```python
from build123d import *

# Parameters (mm, degrees)
SKETCH1_R               = 15.25
SKETCH1_R_2             = 12.75
BOSS_EXTRUDE1_DEPTH     = 4
SKETCH2_R               = 15.25
SKETCH2_R_2             = 7.5
BOSS_EXTRUDE2_DEPTH     = 6
BOSS_EXTRUDE3_START     = -3
SKETCH3_R               = 15.25
BOSS_EXTRUDE3_DEPTH     = 3
SKETCH4_R               = 1.25
CUT_EXTRUDE1_DEPTH      = 10
CUT_EXTRUDE_THIN1_START = -70
CUT_EXTRUDE_THIN1_DEPTH = 25
SKETCH7_R               = 31
SKETCH7_R_2             = 26
BOSS_EXTRUDE4_DEPTH     = 5
CHAMFER3_SIZE           = 3
FILLET3_R               = 1
FILLET4_R               = 10


with BuildPart() as part:
    # Sketch1 → Boss-Extrude1 (new body)
    with BuildSketch(Plane(origin=(0, 0, 0), x_dir=(1, 0, 0), z_dir=(0, 1, 0))):
        with Locations(Location((0, 0, 0), (0, 0, 270))):
            Circle(SKETCH1_R)
        with Locations(Location((0, 0, 0), (0, 0, 270))):
            Circle(SKETCH1_R_2, mode=Mode.SUBTRACT)
    extrude(amount=BOSS_EXTRUDE1_DEPTH)

    # Sketch2 → Boss-Extrude2 (add)
    with BuildSketch(Plane(origin=(0, 4, 0), x_dir=(1, 0, 0), z_dir=(0, 1, 0))):
        with Locations(Location((0, 0, 0), (0, 0, 270))):
            Circle(SKETCH2_R)
        with Locations(Location((0, 0, 0), (0, 0, 270))):
            Circle(SKETCH2_R_2, mode=Mode.SUBTRACT)
    extrude(amount=BOSS_EXTRUDE2_DEPTH)

    # Sketch3 → Boss-Extrude3 (add)
    with BuildSketch(Plane(origin=(0, 10, 0), x_dir=(1, 0, 0), z_dir=(0, 1, 0)).offset(BOSS_EXTRUDE3_START)):
        with Locations(Location((0, 0, 0), (0, 0, 270))):
            Circle(SKETCH3_R)
    extrude(amount=BOSS_EXTRUDE3_DEPTH)

    # Sketch4 → Cut-Extrude1 (cut)
    with BuildSketch(Plane(origin=(0, 4, 0), x_dir=(-1, 0, 0), z_dir=(0, -1, 0))):
        with Locations(Location((5.42938356, -8.987312955, 0), (0, 0, 90))):
            Circle(SKETCH4_R)
        with Locations(Location((-5.068549551, -9.195640568, 0), (0, 0, 90))):
            Circle(SKETCH4_R)
        with Locations(Location((-10.497933111, -0.208327612, 0), (0, 0, 90))):
            Circle(SKETCH4_R)
        with Locations(Location((-5.42938356, 8.987312955, 0), (0, 0, 90))):
            Circle(SKETCH4_R)
        with Locations(Location((5.068549551, 9.195640568, 0), (0, 0, 90))):
            Circle(SKETCH4_R)
        with Locations(Location((10.497933111, 0.208327612, 0), (0, 0, 90))):
            Circle(SKETCH4_R)
    extrude(amount=-CUT_EXTRUDE1_DEPTH, mode=Mode.SUBTRACT)

    # Sketch5 → Revolve1 (revolve)
    with BuildSketch(Plane.XY, mode=Mode.PRIVATE) as revolve1_sk:
        Polygon((-15.25, 0), (-26.2, 0), (-26.2, 20), (-26.2, 40), (-23.2, 40), (-23.2, 21.323043804), (-15.25, 10), align=None)
    revolve(revolve1_sk.sketch.rotate(Axis((0, 0, 0), (0, 1, 0)), 270), axis=Axis((0, 0, 0), (0, 1, 0)))

    # Cut-Extrude-Thin1: read off the stored shape, not the designer's step
    # Cut-Extrude-Thin1 outline → Cut-Extrude-Thin1 (cut)
    with BuildSketch(Plane(origin=(0, 85, 0), x_dir=(1, 0, 0), z_dir=(0, 1, 0)).offset(CUT_EXTRUDE_THIN1_START)):
        with BuildLine():
            Line((1, 1), (1, 26.180909075))
            ThreePointArc((1, 26.180909075), (0, 26.2), (-1, 26.180909075))
            Line((-1, 26.180909075), (-1, 1))
            Line((-1, 1), (1, 1))
        make_face()
        with BuildLine():
            Line((1, 1), (1, -1))
            Line((1, -1), (26.180909075, -1))
            ThreePointArc((26.180909075, -1), (26.2, 0), (26.180909075, 1))
            Line((26.180909075, 1), (1, 1))
        make_face()
        with BuildLine():
            Line((1, -1), (-1, -1))
            Line((-1, -1), (-1, -26.180909075))
            ThreePointArc((-1, -26.180909075), (0, -26.2), (1, -26.180909075))
            Line((1, -26.180909075), (1, -1))
        make_face()
        with BuildLine():
            Line((-1, -1), (-1, 1))
            Line((-1, 1), (-26.180909075, 1))
            ThreePointArc((-26.180909075, 1), (-26.2, 0), (-26.180909075, -1))
            Line((-26.180909075, -1), (-1, -1))
        make_face()
    extrude(amount=CUT_EXTRUDE_THIN1_DEPTH, mode=Mode.SUBTRACT)

    # Sketch7 → Boss-Extrude4 (add)
    with BuildSketch(Plane(origin=(0, 0, 0), x_dir=(-1, 0, 0), z_dir=(0, -1, 0))):
        with Locations(Location((0, 0, 0), (0, 0, 90))):
            Circle(SKETCH7_R)
        Circle(SKETCH7_R_2, mode=Mode.SUBTRACT)
    extrude(amount=-BOSS_EXTRUDE4_DEPTH)

    # Chamfer3
    chamfer3_edges = [part.edges().sort_by_distance(p)[0] for p in [
        (0, 0, 31),
    ]]
    chamfer(chamfer3_edges, length=CHAMFER3_SIZE)

    # Fillet3
    fillet3_edges = [part.edges().sort_by_distance(p)[0] for p in [
        (0, 0, -12.75),
    ]]
    fillet(fillet3_edges, radius=FILLET3_R)

    # Fillet4
    fillet4_edges = [part.edges().sort_by_distance(p)[0] for p in [
        (24.679673666, 40, 1),
        (-24.679673666, 40, -1),
        (-1, 40, 24.679673666),
        (1, 40, -24.679673666),
        (24.679673666, 40, -1),
        (-24.679673666, 40, 1),
        (1, 40, 24.679673666),
        (-1, 40, -24.679673666),
    ]]
    fillet(fillet4_edges, radius=FILLET4_R)


solid = part.part
```
Model file for the job. Use its own axes, mm. A direction names the side the tool comes from. Give positions to 0.01 mm unless a question says otherwise; leave off trailing zeros. Loops run counter-clockwise (first coordinate to the right, second up) from the corner with the lowest first, then second, coordinate; pieces in that order, holes last. Notation, with made-up numbers: (74.25, -3.75) - (132.25, -3.75) arc R8 ccw to (132.25, 8.25) - close; hole circle Ø11 at (32.25, 89.5). An arc over 180 degrees is marked (long way). One line per item, written item: value. Start each with the question number.
1. Slice it at C-C (y = 34). List the corners of the cut face in (x, z), plus the area to 3 significant figures.
2. Slice it at B-B (z = 0). Give the number of separate pieces and of enclosed holes in the cut face, plus the area to 3 significant figures.
3. Slice it at A-A (y = 27). List the corners of the cut face in (x, z).
4. Pull direction Z, two halves, no side cores. Call faces 4 (the cylindrical face through (10.035, 22.255, -24.202)), 5 (the flat face through (24, 21, -1)), 6 (the flat face through (25.4, 5, 7.03)), 7 (the cylindrical face through (9.278, 6.958, 0.479)): pulls with the +Z half, pulls with the -Z half, needs draft (parallel to the pull), parting line crosses it, or undercut.
5. Probe L1, parallel to X at y = 6.15, z = 0; L2, parallel to Z at x = -11, y = 30.5; L3, parallel to X at y = 24, z = -20. List the from-to ranges inside material, lowest first. Write a range as from..to.
6. Which spindle directions (+Z, -Z, +X, -X, +Y, -Y) get a long thin tool onto all of the face, cutting with end or side? Do faces 1 (the flat face through (0, 7, 0)), 2 (the cylindrical face through (-3.85, 36.99, 23.98)), 3 (the flat face through (-24, 21, -1)). Say none if no direction does.
7. Slice it at D-D (x = 0). List the corners of the cut face in (y, z), plus the area to 3 significant figures.
8. Pin check, flat tips, straight feed: pin 1 (6 mm diameter, centred on y = 27, z = -14, fed in from -X); pin 2 (17 mm diameter, centred on x = 0, z = 0, fed in from +Y); pin 3 (24.5 mm diameter, centred on x = -5.5, z = -2.5, fed in from +Y); pin 4 (2 mm diameter, centred on x = 5.43, z = -8.99, fed in from -Y). Stop position of each tip, or through.
Solution:
1. outline: (-26.14, -1.83) arc R26.2 ccw to (-1.83, -26.14) - (-1.83, -23.13) arc R23.2 cw to (-23.13, -1.83) - close; (-26.14, 1.83) - (-23.13, 1.83) arc R23.2 cw to (-1.83, 23.13) - (-1.83, 26.14) arc R26.2 ccw to start; (1.83, -26.14) arc R26.2 ccw to (26.14, -1.83) - (23.13, -1.83) arc R23.2 cw to (1.83, -23.13) - close; (1.83, 23.13) arc R23.2 cw to (23.13, 1.83) - (26.14, 1.83) arc R26.2 ccw to (1.83, 26.14) - close
1. area: 422 mm^2
2. separate pieces: 3
2. enclosed holes: 0
2. area: 478 mm^2
3. outline: (-26.18, -1) arc R26.2 ccw to (-1, -26.18) - (-1, -23.18) arc R23.2 cw to (-23.18, -1) - close; (-26.18, 1) - (-23.18, 1) arc R23.2 cw to (-1, 23.18) - (-1, 26.18) arc R26.2 ccw to start; (1, -26.18) arc R26.2 ccw to (26.18, -1) - (23.18, -1) arc R23.2 cw to (1, -23.18) - close; (1, 23.18) arc R23.2 cw to (23.18, 1) - (26.18, 1) arc R26.2 ccw to (1, 26.18) - close
4. face 4: parting line crosses it
4. face 5: undercut
4. face 6: needs draft
4. face 7: undercut
5. L1: x = -26.2..-11.73, -9.27..-7.5, 7.5..9.27, 11.73..26.2
5. L2: z = -23.78..-20.43, 20.43..23.78
5. L3: x = -16.92..-11.76, 11.76..16.92
6. face 1: -Y
6. face 2: +Z, -Z, +Y
6. face 3: +X, -X, +Y
7. outline: (0, -28) - (3, -31) - (5, -31) - (5, -26.2) - (15, -26.2) - (15, -18.76) - (10, -15.25) - (10, 15.25) - (15, 18.76) - (15, 26.2) - (5, 26.2) - (5, 31) - (3, 31) - (0, 28) - (0, 13.75) arc R1 ccw to (1, 12.75) - (4, 12.75) - (4, 7.5) - (7, 7.5) - (7, -7.5) - (4, -7.5) - (4, -12.75) - (1, -12.75) arc R1 ccw to (0, -13.75) - close
7. area: 508 mm^2
8. pin 1: stops at x = -23.78
8. pin 2: stops at y = 10
8. pin 3: stops at y = 14.33
8. pin 4: passes through
